The figure shows three views and two pictorial views of one solid part (mm, origin at its lowest corner). Answer the questions. Round coordinates to 2 decimals unless told otherwise and drop trailing zeros. Write each loop counter-clockwise with the first axis right and the second up, starting at its lowest first coordinate (ties: lowest second). Pieces come first, ordered by that corner, then holes. Notation, with made-up numbers: (75, 52) - (91, 52) arc R10 cw to (91, 61) - close; hole circle Ø10 at (-33.75, 31.25). An arc over 180 degrees is marked (long way). Answer as CSV lines item,"result". Start each with the question number.
Item 1: Flat-ended cylindrical pins translate along their axes: pin 1 (4 mm diameter, centred on x = 64, y = 6.5, fed in from -Z); pin 2 (23 mm diameter, centred on x = 46.5, z = 41, fed in from +Y). Find the tip coordinate at first contact, or state that the pin passes through.
Item 2: A cutting plane is placed at B-B on x = 72. Determine the outline of the cut face in (y, z), and give its area (3 significant figures).
Item 3: A cutting plane is placed at A-A on z = 50. Determine the outline of the cut face in (x, y), and give its area (3 significant figures).
Item 4: Straight lines are drawn through the part: line 1 along X through (y, z) = (6, 26.5); line 2 along Z through (x, y) = (72, 5.8); line 3 along Y through (x, z) = (47, 43). For each, find the intervals that lie inside material, in ascending order. Write a range as [from, to].
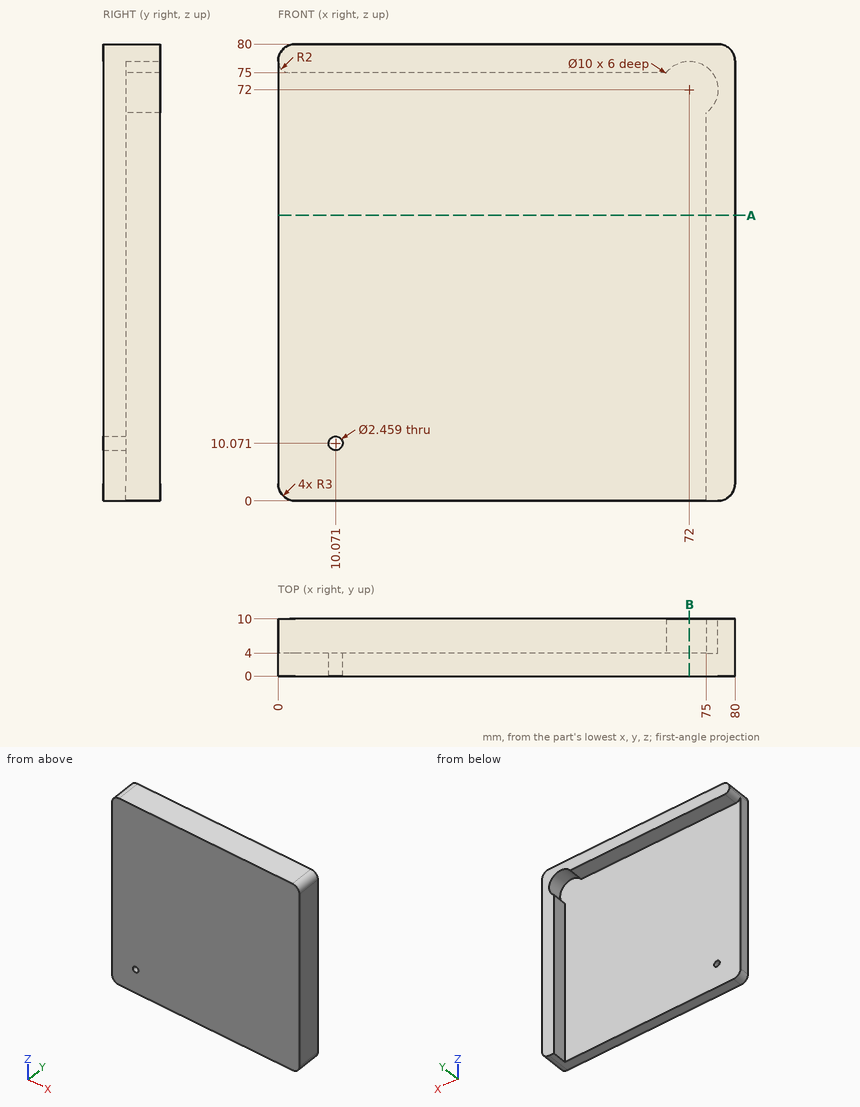
Geometry says:
1,pin 1,"stops at z = 75"
1,pin 2,"stops at y = 4"
2,outline,"(0, 0) - (4, 0) - (4, 77) - (10, 77) - (10, 80) - (0, 80) - close"
2,area,"338 mm^2"
3,outline,"(0, 0) - (80, 0) - (80, 10) - (75, 10) - (75, 4) - (0, 4) - close"
3,area,"350 mm^2"
4,line 1,"x = [75, 80]"
4,line 2,"z = [77, 80]"
4,line 3,"y = [0, 4]"
